CAD build for the part. Positions are in the model's coordinates, mm. A direction names the side the tool comes from. Round coordinates to 2 decimals unless told otherwise and drop trailing zeros. Loops run counter-clockwise (first coordinate to the right, second up) from the corner with the lowest first, then second, coordinate; pieces in that order, holes last.
from build123d import *

# Parameters (mm, degrees)
F0_R     = 3.9
F0_R_2   = 2.7
F1_DEPTH = 20
F2_R     = 2.7
F2_R_2   = 1.95
F3_DEPTH = 1.2
F4_R     = 1.2
F5_R     = 3
F6_DEPTH = 0.8


with BuildPart() as f1:
    # F0 (on Top) → F1 (new body)
    with BuildSketch(Plane.XY):
        Circle(F0_R)
        Circle(F0_R_2, mode=Mode.SUBTRACT)
    extrude(amount=F1_DEPTH)

    # F2 (on face) → F3 (join)
    with BuildSketch(Plane.XY.offset(20)):
        Circle(F2_R)
        Circle(F2_R_2, mode=Mode.SUBTRACT)
    extrude(amount=-F3_DEPTH)

    # F4
    f4_edges = [f1.edges().sort_by_distance(p)[0] for p in [
        (-3.9, 0, 20),
    ]]
    fillet(f4_edges, radius=F4_R)

    # F5 (on face) → F6 (cut)
    with BuildSketch(Plane(origin=(0, 0, 0), x_dir=(1, 0, 0), z_dir=(0, 0, -1))):
        Circle(F5_R)
    extrude(amount=-F6_DEPTH, mode=Mode.SUBTRACT)


solid = f1.part
Item 1: Cut at A-A (x = 0). List the corners of the cut face in (y, z), plus the area to 3 significant figures.
Verdict:
outline: (-3.9, 0) - (-3, 0) - (-3, 0.8) - (-2.7, 0.8) - (-2.7, 18.8) - (-1.95, 18.8) - (-1.95, 20) - (-2.7, 20) arc R1.2 ccw to (-3.9, 18.8) - close; (1.95, 18.8) - (2.7, 18.8) - (2.7, 0.8) - (3, 0.8) - (3, 0) - (3.9, 0) - (3.9, 18.8) arc R1.2 ccw to (2.7, 20) - (1.95, 20) - close
area: 48.7 mm2
Item 2: Cut at C-C (z = 7.75). List the corners of the cut face in (x, y), plus the area to 3 significant figures.
Verdict:
outline: circle Ø7.8 at (0, 0); hole circle Ø5.4 at (0, 0)
area: 24.9 mm2
Item 3: Flat gauge pins, fed straight in: P1, Ø1, axis at x = -2.5, z = 15, coming from the -Y side; P2, Ø1.5, axis at x = -1.5, z = 9, coming from the -Y side; P3, Ø4.5, axis at x = 0, y = 0, coming from the -Z side. Where does each tip first touch, or does it go through?
Verdict:
P1: stops at y = -3.35
P2: stops at y = -3.83
P3: stops at z = 18.8
Item 4: 3-axis set-ups, long thin cutter, end or side, ignore diameter. For faces 4 (the flat face through (1, -2, 18.8)), 5 (the flat face through (1, -3, 0)): which of +Z, -Z, +X, -X, +Y, -Y reach the whole face in a straight line?
Verdict:
face 4: -Z
face 5: -Z, +X, -X, +Y, -Y
Item 5: Wall check: L1, parallel to Y at x = 0, z = 10; L2, parallel to Y at x = 0, z = 0.35; L3, parallel to X at y = -1, z = 9.75. Give the ranges that are in metal, low to high.
Verdict:
L1: y = -3.9 to -2.7, 2.7 to 3.9
L2: y = -3.9 to -3, 3 to 3.9
L3: x = -3.77 to -2.51, 2.51 to 3.77
Item 6: Mould opens along X. For faces 1 (the cylindrical face through (-3, -0.1, 0.4)), 2 (the cylindrical face through (-2.87, 2.64, 9.27)), 3 (the flat face through (1, -2, 20)) say: released by +X, released by -X, zero draft, split by the parting line, or undercut.
Verdict:
face 1: undercut
face 2: split by the parting line
face 3: zero draft
